```python
from build123d import *

# Parameters (mm, degrees)
BOSS_EXTRUDE1_DEPTH = 13
SHELL1_T            = -2
CUT_EXTRUDE1_START  = -2
CUT_EXTRUDE1_DEPTH  = 2
CUT_EXTRUDE2_REACH  = 45.819
SKETCH3_R           = 1.5
SKETCH4_W           = 4
SKETCH4_H           = 4
SKETCH4_R           = 1.5
BOSS_EXTRUDE2_DEPTH = 9
FILLET1_R           = 1


with BuildPart() as part:
    # Sketch1 → Boss-Extrude1 (new body)
    with BuildSketch(Plane(origin=(0, 0, 0), x_dir=(1, 0, 0), z_dir=(0, 1, 0))):
        with BuildLine():
            ThreePointArc((21.75, 17.875), (0, 8.537465971), (-21.75, 17.875))
            Line((-21.75, 17.875), (-21.75, -17.875))
            Line((-21.75, -17.875), (21.75, -17.875))
            Line((21.75, -17.875), (21.75, 17.875))
        make_face()
    extrude(amount=BOSS_EXTRUDE1_DEPTH)

    # Shell1
    shell1_openings = [part.faces().sort_by_distance(p)[0] for p in [
        (0, 13, 3.099956695),
    ]]
    offset(amount=SHELL1_T, openings=shell1_openings, kind=Kind.INTERSECTION)

    # Sketch2 → Cut-Extrude1 (cut)
    with BuildSketch(Plane(origin=(0, 13, 0), x_dir=(1, 0, 0), z_dir=(0, 1, 0)).offset(CUT_EXTRUDE1_START)):
        with BuildLine():
            ThreePointArc((19.75, 15.955670205), (0, 8.537465971), (-19.75, 15.955670205))
            Line((-19.75, 15.955670205), (-19.75, 13.359350474))
            ThreePointArc((-19.75, 13.359350474), (0, 6.537465971), (19.75, 13.359350474))
            Line((19.75, 13.359350474), (19.75, 15.955670205))
        make_face()
    extrude(amount=CUT_EXTRUDE1_DEPTH, mode=Mode.SUBTRACT)

    # Sketch3 → Cut-Extrude2 (cut, up to next)
    with BuildSketch(Plane.XY.offset(17.875), mode=Mode.PRIVATE) as cut_extrude2_sk1:
        with Locations((0, 5)):
            Circle(SKETCH3_R)
    cut_extrude2_tool1 = extrude(cut_extrude2_sk1.sketch, amount=-CUT_EXTRUDE2_REACH, mode=Mode.PRIVATE) & part.part
    add(cut_extrude2_tool1.solids().sort_by_distance((0, 5, 17.875))[0], mode=Mode.SUBTRACT)

    # Sketch4 → Boss-Extrude2 (add)
    with BuildSketch(Plane(origin=(0, 2, 0), x_dir=(1, 0, 0), z_dir=(0, 1, 0))):
        with Locations((17.75, -13.875)):
            Rectangle(SKETCH4_W, SKETCH4_H)
        with Locations(Location((17.75, -13.875, 0), (0, 0, 270))):
            Circle(SKETCH4_R, mode=Mode.SUBTRACT)
    extrude(amount=BOSS_EXTRUDE2_DEPTH)

    # Fillet1
    fillet1_edges = [part.edges().sort_by_distance(p)[0] for p in [
        (15.75, 6.5, 11.875),
    ]]
    fillet(fillet1_edges, radius=FILLET1_R)


solid = part.part
```
Work out the finished part from the listing and answer in its coordinate system (mm). A direction names the side the tool comes from. Round coordinates to 2 decimals unless told otherwise and drop trailing zeros. Order: outer loops, then holes, each group sorted by start corner. A loop starts at its lowest first (then second) coordinate and runs counter-clockwise, first axis right, second up.
Q1. A cutting plane is placed at C-C, the plane z = -2.5. Determine the outline of the cut face in (x, y).
Solution:
outline: (-21.75, 0) - (21.75, 0) - (21.75, 13) - (19.75, 13) - (19.75, 2) - (-19.75, 2) - (-19.75, 13) - (-21.75, 13) - close
Q2. A cutting plane is placed at D-D, the plane y = 11.75. Determine the outline of the cut face in (x, z) (3 decimals), then the cut area to 3 significant figures.
Solution:
outline: (-21.75, -17.875) arc R30 cw to (-19.75, -15.956) - (-19.75, 15.875) - (19.75, 15.875) - (19.75, -15.956) arc R30 cw to (21.75, -17.875) - (21.75, 17.875) - (-21.75, 17.875) - close
area: 218 mm2
Q3. The mould has two halves that part along X. Classify faces 4 (the flat face through (19.75, 7, 0)), 5 (the flat face through (-21.75, 6, 0)), 6 (the flat face through (0, 0, 4)): pulls with the +X half, pulls with the -X half, needs draft (parallel to the pull), parting line crosses it, or undercut.
Solution:
face 4: undercut
face 5: pulls with the -X half
face 6: needs draft
Q4. Find the intervals of material crossed by line 1 along Y through (x, z) = (0, 17.3); line 2 along X through (y, z) = (7, -5.5); line 3 along Z through (x, y) = (17, 6.25) (3 decimals), in increasing order.
Solution:
line 1: y = 0 to 3.5, 6.5 to 13
line 2: x = -21.75 to -19.75, 19.75 to 21.75
line 3: z = -13.819 to -11.427, 11.875 to 12.576, 15.174 to 17.875
Q5. A tool of negligible diameter and unlimited length cuts with its end or side. For faces 1 (the cylindrical face through (-1.5, 5.07, 16.89)), 2 (the flat face through (0, 2, 4)), 3 (the flat face through (19, 11, 15)), from which of +Z, -Z, +X, -X, +Y, -Y can it reach the whole face along a straight path? Write none if from no direction.
Solution:
face 1: +Z
face 2: +Y
face 3: -Z, +Y
Q6. Given pin 1 Ø3 at (x, y) = (-10.5, 4) entering from -Z; pin 2 Ø3 at (x, y) = (14.5, 4.5) entering from -Z; pin 3 Ø3 at (x, z) = (6, -10.5) entering from -Y; pin 4 Ø5.5 at (x, y) = (9, 8.5) entering from -Z, each flat-ended and moving along its own axis, determine where each tip first touches the part or whether it passes through.
Solution:
pin 1: stops at z = -11.04
pin 2: stops at z = -13.16
pin 3: stops at y = 0
pin 4: stops at z = -10.93
Q7. A cutting plane is placed at B-B, the plane y = 5. Determine the outline of the cut face in (x, z) (3 decimals).
Solution:
outline: (-21.75, -17.875) arc R30 cw to (21.75, -17.875) - (21.75, 17.875) - (1.5, 17.875) - (1.5, 15.875) - (15.75, 15.875) - (15.75, 12.875) arc R1 ccw to (16.75, 11.875) - (19.75, 11.875) - (19.75, -13.359) arc R32 ccw to (-19.75, -13.359) - (-19.75, 15.875) - (-1.5, 15.875) - (-1.5, 17.875) - (-21.75, 17.875) - close; hole circle Ø3 at (17.75, 13.875)
Q8. A cutting plane is placed at A-A, the plane x = 0. Determine the outline of the cut face in (y, z) (3 decimals), then the cut area to 3 significant figures.
Solution:
outline: (0, -8.537) - (11, -8.537) - (11, -6.537) - (2, -6.537) - (2, 15.875) - (3.5, 15.875) - (3.5, 17.875) - (0, 17.875) - close; (6.5, 15.875) - (13, 15.875) - (13, 17.875) - (6.5, 17.875) - close
area: 86.8 mm2
